Check sheet for the modelled part. Datum: model origin and axes. Units: mm. A direction names the side the tool comes from. Give positions to 0.01 mm unless a question says otherwise; leave off trailing zeros. Write each loop counter-clockwise with the first axis right and the second up, starting at its lowest first coordinate (ties: lowest second). Pieces come first, ordered by that corner, then holes.
from build123d import *

# Parameters (mm, degrees)
F2_W = 62
F2_H = 10


with BuildPart() as f1:
    # F0 (on Front) → F1 (revolve)
    with BuildSketch(Plane.XZ):
        Polygon((20, 400), (20, 0), (24.15, 0), (24.15, 2000), (21, 2000), (21, 2200), (20, 2200), (20, 1501.37949), align=None)
    revolve(axis=Axis((0, 0, 1100), (0, 0, 1)))

    # F2 (on Front) → F3 (revolve)
    with BuildSketch(Plane.XZ):
        with Locations((31, 395)):
            Rectangle(F2_W, F2_H)
        with Locations((31, 895)):
            Rectangle(F2_W, F2_H)
        with Locations((31, 1395)):
            Rectangle(F2_W, F2_H)
        with Locations((31, 1895)):
            Rectangle(F2_W, F2_H)
    revolve(axis=Axis((0, 0, 197.5), (0, 0, 1)))


solid = f1.part
1) Sectioned sample at B-B on y = 0. Give the number of separate pieces and of enclosed holes in the cut face, then the cut area to 3 significant figures.
2) Sectioned sample at D-D on z = 2068.5. Record the boundary of the cut face in (x, y), then the cut area to 3 significant figures.
3) Sectioned sample at A-A on z = 1190.5. Record the boundary of the cut face in (x, y).
4) Access from +Z, -Z, +X, -X, +Y, -Y to the whole of each face (thin tool, end or side, straight path). Record for faces 1 (the cylindrical face through (-4.336, -19.524, 192.27)), 2 (the cylindrical face through (-4.336, -19.524, 2047.9)), 3 (the flat face through (0, 0, 890)), 4 (the cylindrical face through (-8.071, 61.472, 395.07)).
5) Gauge pin test, flat ends, axial feed: pin 1 (12 mm diameter, centred on x = -9.5, y = 9.5, fed in from -Z); pin 2 (4 mm diameter, centred on x = -34.5, y = 40.5, fed in from +Z); pin 3 (1 mm diameter, centred on x = -2, z = 1368, fed in from +Y). Record the tip position at first contact, or that the pin passes through.
6) Draft check along X on faces 5 (the flat face through (0, 0, 1390)), 6 (the cylindrical face through (-24.127, 1.062, 1950.7)), 7 (the flat face through (1, -27, 1400)), 8 (the flat face through (0, 0, 1890)). Enter one of: +X half, -X half, draft (parallel to the pull), parting line (faces both ways), or undercut.
7) Scan lines: L1, parallel to Z at x = -24.5, y = -37.5; L2, parallel to Y at x = 0, z = 1623.5; L3, parallel to X at y = -1.5, z = 517. Record each from-to range of solid material in increasing order.
Answers below:
1. separate pieces: 1
1. enclosed holes: 3
1. area: 21,600 mm2
2. outline: circle Ø42 at (0, 0); hole circle Ø40 at (0, 0)
2. area: 129 mm2
3. outline: circle Ø48.3 at (0, 0); hole circle Ø40 at (0, 0)
4. face 1: -Z
4. face 2: +Z
4. face 3: none
4. face 4: +Z, -Z
5. pin 1: stops at z = 390
5. pin 2: stops at z = 1900
5. pin 3: stops at y = 24.1
6. face 5: undercut
6. face 6: parting line
6. face 7: draft
6. face 8: undercut
7. L1: z = 390 to 400, 890 to 900, 1390 to 1400, 1890 to 1900
7. L2: y = -24.15 to -20, 20 to 24.15
7. L3: x = -24.1 to -19.94, 19.94 to 24.1
